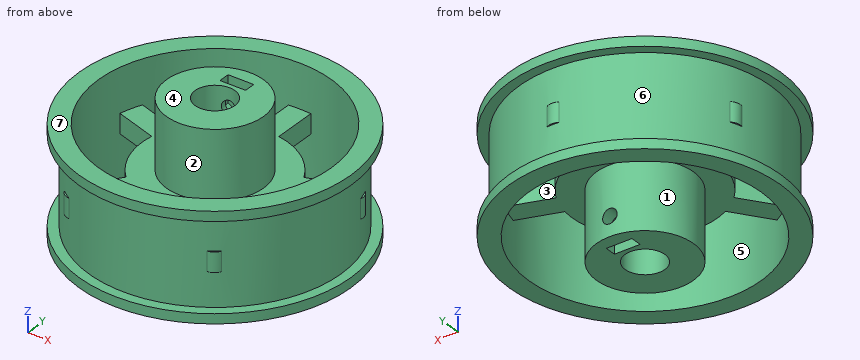
```python
from build123d import *

# Parameters (mm, degrees)
BOSS_EXTRUDE1_DEPTH      = 2
BOSS_EXTRUDE1_DEPTH_BACK = 2
SKETCH3_R                = 15
BOSS_EXTRUDE2_DEPTH      = 16
BOSS_EXTRUDE2_DEPTH_BACK = 16
SKETCH6_R                = 10
CUT_EXTRUDE6_DEPTH       = 43.670158732
CUT_EXTRUDE6_DEPTH_BACK  = 43.670158732
SKETCH7_R                = 4.1
BOSS_EXTRUDE3_DEPTH      = 2
BOSS_EXTRUDE3_DEPTH_BACK = 2
SKETCH10_W               = 5.3
SKETCH10_H               = 2.3
CUT_EXTRUDE7_DEPTH       = 4
CUT_EXTRUDE8_START       = -4
SKETCH11_R               = 1.5
CUT_EXTRUDE8_DEPTH       = 10
CUT_EXTRUDE9_DEPTH       = 2.3


with BuildPart() as part:
    # Sketch2 → Revolve1 (revolve)
    with BuildSketch(Plane(origin=(0, 0, 0), x_dir=(0, 0, -1), z_dir=(1, 0, 0)), mode=Mode.PRIVATE) as revolve1_sk:
        Polygon((-9, 25.970899576), (9, 25.970899576), (9, 27.970899576), (11, 27.970899576), (11, 23.970899576), (-11, 23.970899576), (-11, 27.970899576), (-9, 27.970899576), align=None)
    revolve(revolve1_sk.sketch.rotate(Axis((0, 0, 10), (0, 0, -1)), 90), axis=Axis((0, 0, 10), (0, 0, -1)))



with BuildPart() as body_2:
    # Sketch3 → Boss-Extrude1 (new, two sides: drawn at the far end of the back side and taken through both)
    with BuildSketch(Plane.XY.offset(-BOSS_EXTRUDE1_DEPTH_BACK)):
        Circle(SKETCH3_R)
    extrude(amount=BOSS_EXTRUDE1_DEPTH + BOSS_EXTRUDE1_DEPTH_BACK)

    # Sketch6 → Boss-Extrude2 (add, two sides: drawn at the far end of the back side and taken through both)
    with BuildSketch(Plane.XY.offset(-BOSS_EXTRUDE2_DEPTH_BACK)):
        Circle(SKETCH6_R)
    extrude(amount=BOSS_EXTRUDE2_DEPTH + BOSS_EXTRUDE2_DEPTH_BACK)

    # Sketch7 → Cut-Extrude6 (cut, two sides: drawn at the far end of the back side and taken through both)
    with BuildSketch(Plane.XY.offset(-CUT_EXTRUDE6_DEPTH_BACK)):
        Circle(SKETCH7_R)
    extrude(amount=CUT_EXTRUDE6_DEPTH + CUT_EXTRUDE6_DEPTH_BACK, mode=Mode.SUBTRACT)


with BuildPart() as part_1:
    add(part.part)

    add(body_2.part)  # Boss-Extrude3 merges body 2
    # Sketch8 → Boss-Extrude3 (add, two sides: drawn at the far end of the back side and taken through both)
    with BuildSketch(Plane.XY.offset(-BOSS_EXTRUDE3_DEPTH_BACK)):
        with BuildLine():
            Line((-2.314963667, 11.983341333), (-2.314963667, 23.970899576))
            ThreePointArc((-2.314963667, 23.970899576), (0, 26.285863243), (2.314963667, 23.970899576))
            Line((2.314963667, 23.970899576), (2.314963667, 11.983341333))
            ThreePointArc((2.314963667, 11.983341333), (0, 9.668377666), (-2.314963667, 11.983341333))
        make_face()
        with BuildLine():
            Line((10.681471747, 5.904717401), (22.082317129, 9.60907662))
            ThreePointArc((22.082317129, 9.60907662), (24.999341523, 8.122778454), (23.513043358, 5.205754059))
            Line((23.513043358, 5.205754059), (12.112197976, 1.501394841))
            ThreePointArc((12.112197976, 1.501394841), (9.195173582, 2.987693007), (10.681471747, 5.904717401))
        make_face()
        with BuildLine():
            Line((8.916476256, -8.334025285), (15.962586203, -18.032163625))
            ThreePointArc((15.962586203, -18.032163625), (15.450442758, -21.265710075), (12.216896307, -20.75356663))
            Line((12.216896307, -20.75356663), (5.170786361, -11.055428291))
            ThreePointArc((5.170786361, -11.055428291), (5.682929806, -7.82188184), (8.916476256, -8.334025285))
        make_face()
        with BuildLine():
            Line((-5.170786361, -11.055428291), (-12.216896307, -20.75356663))
            ThreePointArc((-12.216896307, -20.75356663), (-15.450442758, -21.265710075), (-15.962586203, -18.032163625))
            Line((-15.962586203, -18.032163625), (-8.916476256, -8.334025285))
            ThreePointArc((-8.916476256, -8.334025285), (-5.682929806, -7.82188184), (-5.170786361, -11.055428291))
        make_face()
        with BuildLine():
            Line((-12.112197976, 1.501394841), (-23.513043358, 5.205754059))
            ThreePointArc((-23.513043358, 5.205754059), (-24.999341523, 8.122778454), (-22.082317129, 9.60907662))
            Line((-22.082317129, 9.60907662), (-10.681471747, 5.904717401))
            ThreePointArc((-10.681471747, 5.904717401), (-9.195173582, 2.987693007), (-12.112197976, 1.501394841))
        make_face()
    extrude(amount=BOSS_EXTRUDE3_DEPTH + BOSS_EXTRUDE3_DEPTH_BACK)

    # Sketch10 → Cut-Extrude7 (cut)
    with BuildSketch(Plane.XY.offset(12)):
        with Locations((0, 6.15)):
            Rectangle(SKETCH10_W, SKETCH10_H)
    cut_extrude7 = extrude(amount=CUT_EXTRUDE7_DEPTH, mode=Mode.SUBTRACT)

    # Sketch11 → Cut-Extrude8 (cut)
    with BuildSketch(Plane(origin=(0, 5, 0), x_dir=(1, 0, 0), z_dir=(0, 1, 0)).offset(CUT_EXTRUDE8_START)):
        with Locations((0, -12)):
            Circle(SKETCH11_R)
    cut_extrude8 = extrude(amount=CUT_EXTRUDE8_DEPTH, mode=Mode.SUBTRACT)

    # Sketch12 → Cut-Extrude9 (cut)
    with BuildSketch(Plane(origin=(0, 5, 0), x_dir=(1, 0, 0), z_dir=(0, 1, 0))):
        Polygon((0, -15.059956427), (2.65, -13.529978213), (2.65, -10.470021787), (0, -8.940043573), (-2.65, -10.470021787), (-2.65, -13.529978213), align=None)
    cut_extrude9 = extrude(amount=CUT_EXTRUDE9_DEPTH, mode=Mode.SUBTRACT)

    # Mirror1: Cut-Extrude7, Cut-Extrude8, Cut-Extrude9 across plane
    add(cut_extrude7.mirror(Plane.XY), mode=Mode.SUBTRACT)
    add(cut_extrude8.mirror(Plane.XY), mode=Mode.SUBTRACT)
    add(cut_extrude9.mirror(Plane.XY), mode=Mode.SUBTRACT)


solid = part_1.part
```
Here's how the part is built. I have some questions about the finished solid (model axes, mm). Face numbers are marked on the shaded views. A direction names the side the tool comes from. Round coordinates to 2 decimals unless told otherwise and drop trailing zeros. Loops run counter-clockwise (first coordinate to the right, second up) from the corner with the lowest first, then second, coordinate; pieces in that order, holes last.
1. Suppose I cut it at B-B, the plane z = 5.5. Please give me the cut outline in (x, y), and give its area (3 significant figures).
Answers:
outline: circle Ø51.94 at (0, 0); circle Ø20 at (0, 0); hole circle Ø47.94 at (0, 0); hole circle Ø8.2 at (0, 0)
area: 575 mm2
2. If I drill on probe 1 along Y at (x, z) = (0, 4); probe 2 along Z at (x, y) = (0, 8); probe 3 along X at (y, z) = (4.5, -12), over which ranges is the centre line in solid material (lowest first)?
Answers:
probe 1: y = -25.97 to -23.97, -10 to -4.1, 4.1 to 10, 23.97 to 25.97
probe 2: z = -16 to -13.5, -10.5 to 10.5, 13.5 to 16
probe 3: x = -8.93 to -1.5, 1.5 to 8.93
3. Thinking about a two-plate mould opening in Y: for the marked faces 5, 6 and 7, which applies, released by +Y, released by -Y, zero draft, split by the parting line, or undercut?
Answers:
face 5: undercut
face 6: split by the parting line
face 7: zero draft
4. Suppose I cut it at A-A, the plane y = 0. Give the number of separate pieces and of enclosed holes in the cut face, and give its area (3 significant figures).
Answers:
separate pieces: 4
enclosed holes: 0
area: 522 mm2
5. For the marked faces 1, 2, 3 and 4, which set-ups out of +Z, -Z, +X, -X, +Y, -Y let a thin tool reach every point of the face, with its end or its side?
Answers:
face 1: -Z
face 2: +Z
face 3: +Z, -Z
face 4: +Z, +X, -X, +Y, -Y
6. Will these pins go through, and if not, where does the flat tip stop? pin 1 (1 mm diameter, centred on x = -15, y = -9, fed in from +Z); pin 2 (5 mm diameter, centred on x = 15.5, z = 7.5, fed in from +Y); pin 3 (1.6 mm diameter, centred on x = 15.5, y = -20.5, fed in from +Z); pin 4 (0.7 mm diameter, centred on x = 15.5, y = -20.5, fed in from -Z).
Answers:
pin 1: passes through
pin 2: stops at y = 24.5
pin 3: stops at z = 11
pin 4: stops at z = -11
7. Suppose I cut it at C-C, the plane y = 22. Please give me the cut outline in (x, z), and give its area (3 significant figures).
Answers:
outline: (-17.27, -11) - (-9.52, -11) - (-9.52, 11) - (-17.27, 11) - (-17.27, 9) - (-13.8, 9) - (-13.8, -9) - (-17.27, -9) - close; (-2.31, -2) - (2.31, -2) - (2.31, 2) - (-2.31, 2) - close; (9.52, -11) - (17.27, -11) - (17.27, -9) - (13.8, -9) - (13.8, 9) - (17.27, 9) - (17.27, 11) - (9.52, 11) - close
area: 235 mm2
